Verification items for the finished model (mm, model axes). A direction names the side the tool comes from. Give positions to 0.01 mm unless a question says otherwise; leave off trailing zeros. Loops run counter-clockwise (first coordinate to the right, second up) from the corner with the lowest first, then second, coordinate; pieces in that order, holes last. Notation, with made-up numbers: (79, -8) - (92, -8) arc R29 cw to (92, 13) - close; hole circle Ø11 at (10.25, 35). An arc over 180 degrees is marked (long way). One line per question, with ' | ' between items. Start each with the question number.
1. Thickness scan on line 1 along Y through (x, z) = (53, -7); line 2 along X through (y, z) = (-22, -8); line 3 along X through (y, z) = (-9.5, 90). Record the ranges inside material, lowest first. Write a range as from..to.
2. Tool access check on faces 4 (the face through (-19.05, 0, 56)), 5 (the face through (23.59, 23.49, 102.58)), 6 (the face through (-6, -30, 155)), 7 (the face through (0, -25.4, 74)), 8 (the face through (-6, 30, 155)). Record the directions out of +Z, -Z, +X, -X, +Y, -Y that give a thin tool (end or side, any length) a straight path to the whole face; none if there is none.
3. Section check D-D, the plane y = 22.5. Enter the section's corners in (x, z), then the cut area to 3 significant figures.
4. Depth check by flat-ended pin: pin 1 Ø20.5 at (x, z) = (6, 78.5) entering from +Y; pin 2 Ø19 at (x, y) = (-53, -22.5) entering from +Z; pin 3 Ø7.5 at (y, z) = (0.5, 71.5) entering from -X; pin 4 Ø11 at (x, y) = (53, 22.5) entering from +Z. Enter the tip coordinate at first touch or a pass-through.
5. Mould release check, pull along Z, two halves, no side actions. Record for faces 1 (the face through (21.05, 0.42, 212.76)), 2 (the face through (25.4, 0, 103)), 3 (the face through (65, -1, -6)): +Z half, -Z half, draft (parallel to the pull), parting line (faces both ways), or undercut.
6. Section check B-B, the plane z = 2.5. Enter the section's corners in (x, y), then the cut area to 3 significant figures.
7. Section check C-C, the plane x = -53. Enter the section's corners in (y, z), then the cut area to 3 significant figures.
8. Section check A-A, the plane y = 0.5. Enter the section's corners in (x, z), then the cut area to 3 significant figures.
from build123d import *

# Parameters (mm, degrees)
F0_W     = 130
F0_H     = 75
F1_DEPTH = 12
F3_DEPTH = 208.083
F5_D     = 12
F7_DEPTH = 50.8
F8_W     = 60
F8_H     = 125
F9_DEPTH = 12


with BuildPart() as f1:
    # F0 (on Top) → F1 (new body)
    with BuildSketch(Plane.XY):
        Rectangle(F0_W, F0_H)
    extrude(amount=-F1_DEPTH)

    # F2 (on face) → F3 (join)
    with BuildSketch(Plane.XY):
        with BuildLine():
            Line((-19.05, -25.4), (19.05, -25.4))
            ThreePointArc((19.05, -25.4), (23.5401280605, -23.5401280605), (25.4, -19.05))
            Line((25.4, -19.05), (25.4, 19.05))
            ThreePointArc((25.4, 19.05), (23.5401280605, 23.5401280605), (19.05, 25.4))
            Line((19.05, 25.4), (-19.05, 25.4))
            ThreePointArc((-19.05, 25.4), (-23.5401280605, 23.5401280605), (-25.4, 19.05))
            Line((-25.4, 19.05), (-25.4, -19.05))
            ThreePointArc((-25.4, -19.05), (-23.5401280605, -23.5401280605), (-19.05, -25.4))
        make_face()
        with BuildLine():
            Line((-12.7, 19.05), (12.7, 19.05))
            ThreePointArc((12.7, 19.05), (17.1901280605, 17.1901280605), (19.05, 12.7))
            Line((19.05, 12.7), (19.05, -12.7))
            ThreePointArc((19.05, -12.7), (17.1901280605, -17.1901280605), (12.7, -19.05))
            Line((12.7, -19.05), (-12.7, -19.05))
            ThreePointArc((-12.7, -19.05), (-17.1901280605, -17.1901280605), (-19.05, -12.7))
            Line((-19.05, -12.7), (-19.05, 12.7))
            ThreePointArc((-19.05, 12.7), (-17.1901280605, 17.1901280605), (-12.7, 19.05))
        make_face(mode=Mode.SUBTRACT)
    extrude(amount=F3_DEPTH)

    # F5 (through all)
    with Locations(Plane.XY):
        with Locations((-53, 22.5), (53, 22.5), (53, -22.5), (-53, -22.5)):
            Hole(F5_D / 2)

    # F6 (on face) → F7 (cut)
    with BuildSketch(Plane.XZ.offset(25.4)):
        Polygon((19.05, 208.083), (-19.05, 208.083), (-19.05, 112.7596673834), (19.05, 194.4653810548), align=None)
        Polygon((25.4, 208.083), (19.05, 208.083), (19.05, 194.4653810548), align=None)
        Polygon((-19.05, 112.7596673834), (-19.05, 208.083), (-25.4, 208.083), (-25.4, 99.1420484381), align=None)
    extrude(amount=-F7_DEPTH, mode=Mode.SUBTRACT)

    # F8 (on face) → F9 (join)
    with BuildSketch(Plane(origin=(-58.8370102857, 0, 27.4361484792), x_dir=(0, -1, 0), z_dir=(-0.906307787, 0, 0.4226182617))):
        with Locations((0, 139.2202268861)):
            Rectangle(F8_W, F8_H)
        with BuildLine():
            Line((25.4, 184.2963670451), (25.4, 94.144086727))
            add(Edge.make_bspline(
                [(25.4, 94.144086727), (25.4, 79.118706674), (19.05, 79.118706674)],
                knots=[4.7123889804, 4.7123889804, 4.7123889804, 6.2831853072, 6.2831853072, 6.2831853072], degree=2, weights=[1, 0.7071067812, 1]))
            Line((19.05, 79.118706674), (-19.05, 79.118706674))
            add(Edge.make_bspline(
                [(-19.05, 79.118706674), (-25.4, 79.118706674), (-25.4, 94.144086727)],
                knots=[0, 0, 0, 1.5707963268, 1.5707963268, 1.5707963268], degree=2, weights=[1, 0.7071067812, 1]))
            Line((-25.4, 94.144086727), (-25.4, 184.2963670451))
            add(Edge.make_bspline(
                [(-25.4, 184.2963670451), (-25.4, 199.3217470982), (-19.05, 199.3217470982)],
                knots=[1.5707963268, 1.5707963268, 1.5707963268, 3.1415926536, 3.1415926536, 3.1415926536], degree=2, weights=[1, 0.7071067812, 1]))
            Line((-19.05, 199.3217470982), (19.05, 199.3217470982))
            add(Edge.make_bspline(
                [(19.05, 199.3217470982), (25.4, 199.3217470982), (25.4, 184.2963670451)],
                knots=[3.1415926536, 3.1415926536, 3.1415926536, 4.7123889804, 4.7123889804, 4.7123889804], degree=2, weights=[1, 0.7071067812, 1]))
        make_face(mode=Mode.SUBTRACT)
        with BuildLine():
            add(Edge.make_bspline(
                [(25.4, 94.144086727), (25.4, 79.118706674), (19.05, 79.118706674)],
                knots=[4.7123889804, 4.7123889804, 4.7123889804, 6.2831853072, 6.2831853072, 6.2831853072], degree=2, weights=[1, 0.7071067812, 1]))
            Line((25.4, 94.144086727), (25.4, 184.2963670451))
            add(Edge.make_bspline(
                [(19.05, 199.3217470982), (25.4, 199.3217470982), (25.4, 184.2963670451)],
                knots=[3.1415926536, 3.1415926536, 3.1415926536, 4.7123889804, 4.7123889804, 4.7123889804], degree=2, weights=[1, 0.7071067812, 1]))
            Line((19.05, 199.3217470982), (-19.05, 199.3217470982))
            add(Edge.make_bspline(
                [(-25.4, 184.2963670451), (-25.4, 199.3217470982), (-19.05, 199.3217470982)],
                knots=[1.5707963268, 1.5707963268, 1.5707963268, 3.1415926536, 3.1415926536, 3.1415926536], degree=2, weights=[1, 0.7071067812, 1]))
            Line((-25.4, 184.2963670451), (-25.4, 94.144086727))
            add(Edge.make_bspline(
                [(-19.05, 79.118706674), (-25.4, 79.118706674), (-25.4, 94.144086727)],
                knots=[0, 0, 0, 1.5707963268, 1.5707963268, 1.5707963268], degree=2, weights=[1, 0.7071067812, 1]))
            Line((-19.05, 79.118706674), (19.05, 79.118706674))
        make_face()
        with BuildLine():
            Line((12.7, 94.144086727), (-12.7, 94.144086727))
            add(Edge.make_bspline(
                [(-12.7, 94.144086727), (-19.05, 94.144086727), (-19.05, 109.1694667801)],
                knots=[0, 0, 0, 1.5707963268, 1.5707963268, 1.5707963268], degree=2, weights=[1, 0.7071067812, 1]))
            Line((-19.05, 109.1694667801), (-19.05, 169.2709869921))
            add(Edge.make_bspline(
                [(-19.05, 169.2709869921), (-19.05, 184.2963670451), (-12.7, 184.2963670451)],
                knots=[1.5707963268, 1.5707963268, 1.5707963268, 3.1415926536, 3.1415926536, 3.1415926536], degree=2, weights=[1, 0.7071067812, 1]))
            Line((-12.7, 184.2963670451), (12.7, 184.2963670451))
            add(Edge.make_bspline(
                [(12.7, 184.2963670451), (19.05, 184.2963670451), (19.05, 169.2709869921)],
                knots=[3.1415926536, 3.1415926536, 3.1415926536, 4.7123889804, 4.7123889804, 4.7123889804], degree=2, weights=[1, 0.7071067812, 1]))
            Line((19.05, 169.2709869921), (19.05, 109.1694667801))
            add(Edge.make_bspline(
                [(19.05, 109.1694667801), (19.05, 94.144086727), (12.7, 94.144086727)],
                knots=[4.7123889804, 4.7123889804, 4.7123889804, 6.2831853072, 6.2831853072, 6.2831853072], degree=2, weights=[1, 0.7071067812, 1]))
        make_face(mode=Mode.SUBTRACT)
        with BuildLine():
            add(Edge.make_bspline(
                [(-12.7, 94.144086727), (-19.05, 94.144086727), (-19.05, 109.1694667801)],
                knots=[0, 0, 0, 1.5707963268, 1.5707963268, 1.5707963268], degree=2, weights=[1, 0.7071067812, 1]))
            Line((-12.7, 94.144086727), (12.7, 94.144086727))
            add(Edge.make_bspline(
                [(19.05, 109.1694667801), (19.05, 94.144086727), (12.7, 94.144086727)],
                knots=[4.7123889804, 4.7123889804, 4.7123889804, 6.2831853072, 6.2831853072, 6.2831853072], degree=2, weights=[1, 0.7071067812, 1]))
            Line((19.05, 109.1694667801), (19.05, 169.2709869921))
            add(Edge.make_bspline(
                [(12.7, 184.2963670451), (19.05, 184.2963670451), (19.05, 169.2709869921)],
                knots=[3.1415926536, 3.1415926536, 3.1415926536, 4.7123889804, 4.7123889804, 4.7123889804], degree=2, weights=[1, 0.7071067812, 1]))
            Line((12.7, 184.2963670451), (-12.7, 184.2963670451))
            add(Edge.make_bspline(
                [(-19.05, 169.2709869921), (-19.05, 184.2963670451), (-12.7, 184.2963670451)],
                knots=[1.5707963268, 1.5707963268, 1.5707963268, 3.1415926536, 3.1415926536, 3.1415926536], degree=2, weights=[1, 0.7071067812, 1]))
            Line((-19.05, 169.2709869921), (-19.05, 109.1694667801))
        make_face()
    extrude(amount=F9_DEPTH)


solid = f1.part
Results list:
1) line 1: -37.5..-28.5, -16.5..16.5, 28.5..37.5 | line 2: -65..-58.98, -47.02..47.02, 58.98..65 | line 3: -25.4..-19.05, 19.05..25.4
2) face 4: none | face 5: +X, +Y | face 6: +Z, +X, -X, -Y | face 7: +X, -Y | face 8: +Z, +X, -X, +Y
3) outline: (-65, -12) - (-59, -12) - (-59, 0) - (-65, 0) - close; (-47, -12) - (47, -12) - (47, 0) - (24.38, 0) - (24.38, 205.9) - (26.41, 210.26) - (15.54, 215.33) - (-37.29, 102.04) - (-26.41, 96.97) - (-24.38, 101.33) - (-24.38, 0) - (-47, 0) - close; (59, -12) - (65, -12) - (65, 0) - (59, 0) - close | area: 10,300 mm²
4) pin 1: y = 25.4 | pin 2: z = 0 | pin 3: x = -25.4 | pin 4: through
5) face 1: +Z half | face 2: undercut | face 3: draft
6) outline: (-25.4, -19.05) arc R6.35 ccw to (-19.05, -25.4) - (19.05, -25.4) arc R6.35 ccw to (25.4, -19.05) - (25.4, 19.05) arc R6.35 ccw to (19.05, 25.4) - (-19.05, 25.4) arc R6.35 ccw to (-25.4, 19.05) - close; hole (-19.05, -12.7) arc R6.35 ccw to (-12.7, -19.05) - (12.7, -19.05) arc R6.35 ccw to (19.05, -12.7) - (19.05, 12.7) arc R6.35 ccw to (12.7, 19.05) - (-12.7, 19.05) arc R6.35 ccw to (-19.05, 12.7) - close | area: 1,130 mm²
7) outline: (-37.5, -12) - (-28.5, -12) - (-28.5, 0) - (-37.5, 0) - close; (-16.5, -12) - (16.5, -12) - (16.5, 0) - (-16.5, 0) - close; (28.5, -12) - (37.5, -12) - (37.5, 0) - (28.5, 0) - close | area: 612 mm²
8) outline: (-65, -12) - (65, -12) - (65, 0) - (25.4, 0) - (25.4, 208.08) - (26.41, 210.26) - (15.54, 215.33) - (-37.29, 102.04) - (-26.41, 96.97) - (-25.4, 99.14) - (-25.4, 0) - (-65, 0) - close; hole (-19.05, 0) - (19.05, 0) - (19.05, 194.47) - (-19.05, 112.76) - close | area: 5,010 mm²
